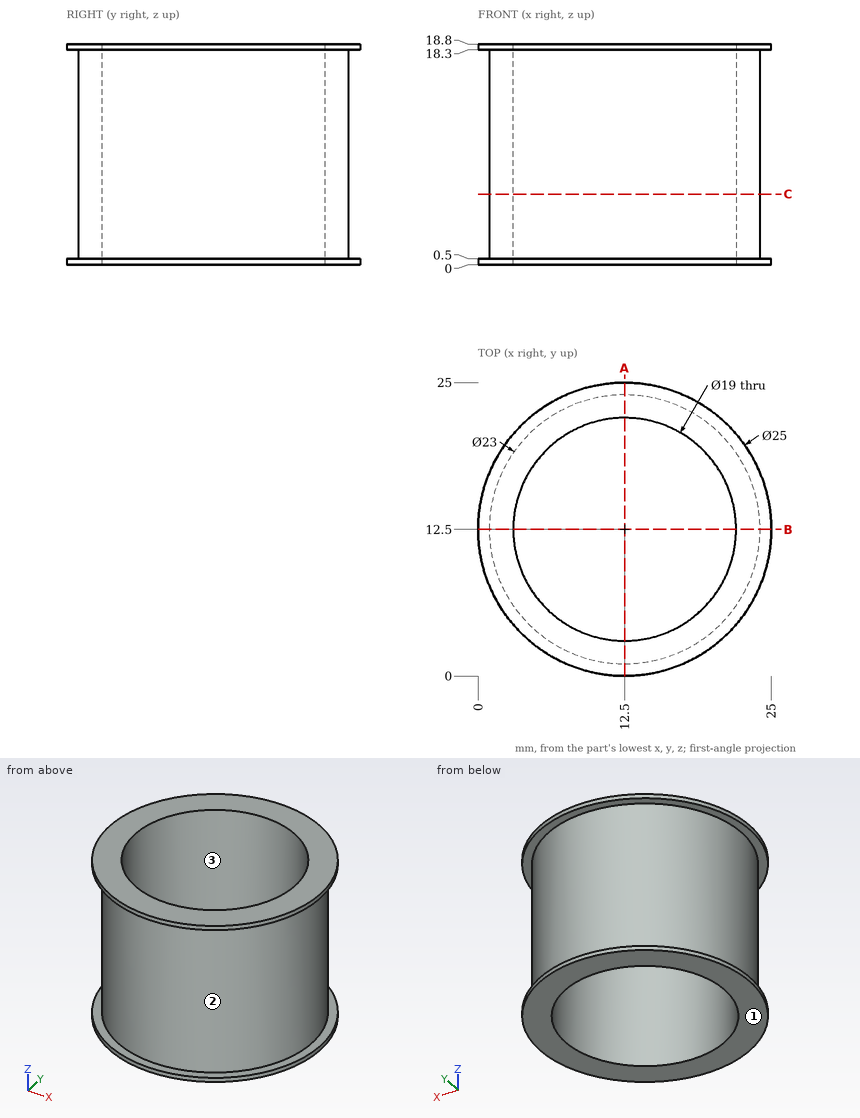
The drawing under review shows one solid part. Ordinate dimensions are in mm from its lowest x, y, z. Round coordinates to 2 decimals unless told otherwise and drop trailing zeros. Order: outer loops, then holes, each group sorted by start corner. A loop starts at its lowest first (then second) coordinate and runs counter-clockwise, first axis right, second up. Notation, with made-up numbers: (-13.75, -28.75) -> (11.25, -28.75) arc R30 ccw to (11.25, -6.75) -> close; hole circle Ø11 at (5, 57.25). An arc over 180 degrees is marked (long way). Use a Markdown table: item, result.
Q1. We need section C-C on z = 6. Write out the cut boundary in (x, y), then the cut area to 3 significant figures.
Values:
| item | result |
|---|---|
| outline | circle Ø23 at (12.5, 12.5); hole circle Ø19 at (12.5, 12.5) |
| area | 132 mm^2 |
Q2. We need section A-A on x = 12.5. Write out the cut boundary in (y, z), then the cut area to 3 significant figures.
Values:
| item | result |
|---|---|
| outline | (0, 0) -> (3, 0) -> (3, 18.8) -> (0, 18.8) -> (0, 18.3) -> (1, 18.3) -> (1, 0.5) -> (0, 0.5) -> close; (22, 0) -> (25, 0) -> (25, 0.5) -> (24, 0.5) -> (24, 18.3) -> (25, 18.3) -> (25, 18.8) -> (22, 18.8) -> close |
| area | 77.2 mm^2 |
Q3. Mouldability with a two-part tool opening along Z and no side actions: class the marked faces 1, 2 and 3 as +Z half, -Z half, draft (parallel to the pull), parting line (faces both ways), or undercut.
Values:
| item | result |
|---|---|
| face 1 | -Z half |
| face 2 | undercut |
| face 3 | draft |
Q4. For line 1 (Y direction, x = 12.5, z = 10); line 2 (Z direction, x = 19.5, y = 22.75); line 3 (X direction, y = 5, z = 14.5), list the stretches that pass through material, from the lowest coordinate up.
Values:
| item | result |
|---|---|
| line 1 | y = 1 to 3, 22 to 24 |
| line 2 | z = 0 to 0.5, 18.3 to 18.8 |
| line 3 | x = 3.78 to 6.67, 18.33 to 21.22 |
Q5. Clearance check with flat-ended pins moving along their axes: P1, Ø4, axis at y = 5.5, z = 6, coming from the -X side; P2, Ø1.5, axis at y = 16, z = 6.5, coming from the -X side; P3, Ø4, axis at x = 14, z = 13, coming from the +Y side. State where each tip first meets the part, or that it passes through.
Values:
| item | result |
|---|---|
| P1 | stops at x = 2.14 |
| P2 | stops at x = 1.33 |
| P3 | stops at y = 24 |
